```python
from build123d import *

# Parameters (mm, degrees)
SM_BASE_FLANGE_1_DEPTH = 765.5
HOLE_WIZARD_M6_1_D     = 7
HOLE_WIZARD_M5_1_D     = 4.2
HOLE_WIZARD_1_D        = 57


# Sheet-metal steps are written as plain solids
with BuildPart() as part:
    # Sketch 1 → 基体-法兰1 (new, symmetric)
    with BuildSketch(Plane(origin=(0, 0, 0), x_dir=(0, 0, -1), z_dir=(1, 0, 0))):
        with BuildLine():
            Line((0, 0), (0, 17.5))
            ThreePointArc((0, 17.5), (0.732233047, 19.267766953), (2.5, 20))
            Line((2.5, 20), (119, 20))
            ThreePointArc((119, 20), (119.707106781, 20.292893219), (120, 21))
            Line((120, 21), (120, 30))
            Line((120, 30), (121.5, 30))
            Line((121.5, 30), (121.5, 21))
            ThreePointArc((121.5, 21), (120.767766953, 19.232233047), (119, 18.5))
            Line((119, 18.5), (2.5, 18.5))
            ThreePointArc((2.5, 18.5), (1.792893219, 18.207106781), (1.5, 17.5))
            Line((1.5, 17.5), (1.5, 0))
            Line((1.5, 0), (0, 0))
        make_face()
    extrude(amount=SM_BASE_FLANGE_1_DEPTH, both=True)

    # M6 间隙孔1 (through all)
    with Locations(Plane(origin=(0, 0, -1.5), x_dir=(-1, 0, 0), z_dir=(0, 0, -1))):
        with Locations((-650, 8), (0, 8), (650, 8)):
            Hole(HOLE_WIZARD_M6_1_D / 2)

    # M5 螺纹孔1 (through all)
    with Locations(Plane(origin=(0, 20, 0), x_dir=(1, 0, 0), z_dir=(0, 1, 0))):
        with Locations((645.5, 36), (623, 36), (623, 101), (645.5, 101)):
            Hole(HOLE_WIZARD_M5_1_D / 2)

    # 孔1 (through all)
    with Locations(Plane(origin=(0, 20, 0), x_dir=(1, 0, 0), z_dir=(0, 1, 0))):
        with Locations((730.5, 68.5)):
            Hole(HOLE_WIZARD_1_D / 2)


solid = part.part
```
Could you check a few things on this model? Use its own coordinates, in mm. Coordinates: 2 decimals unless noted, no trailing zeros. Write each loop counter-clockwise with the first axis right and the second up, starting at its lowest first coordinate (ties: lowest second). Pieces come first, ordered by that corner, then holes. Notation, with made-up numbers: (72, 36) - (116, 36) arc R12 ccw to (116, 59) - close; hole circle Ø1 at (18.5, 77). An arc over 180 degrees is marked (long way). Use a Markdown table: item, result.
Q1. Please list where these lines run through material, in increasing order: L1, parallel to X at y = 19.4, z = -36; L2, parallel to Z at x = 645.5, y = 19.65; L3, parallel to X at y = 18.85, z = -68.5.
Geometry check:
| item | result |
|---|---|
| L1 | x = -765.5 to 620.9, 625.1 to 643.4, 647.6 to 765.5 |
| L2 | z = -121.1 to -103.1, -98.9 to -38.1, -33.9 to -1.22 |
| L3 | x = -765.5 to 702, 759 to 765.5 |
Q2. Imagine slicing it at C-C (x = 207.5). List the corners of the cut face in (y, z) for me, and give its area (3 significant figures).
Geometry check:
| item | result |
|---|---|
| outline | (0, -1.5) - (17.5, -1.5) arc R1 cw to (18.5, -2.5) - (18.5, -119) arc R2.5 ccw to (21, -121.5) - (30, -121.5) - (30, -120) - (21, -120) arc R1 cw to (20, -119) - (20, -2.5) arc R2.5 ccw to (17.5, 0) - (0, 0) - close |
| area | 223 mm2 |
Q3. I'm going to push flat-ended pins straight in: pin 1 Ø3 at (x, z) = (48, -21) entering from -Y; pin 2 Ø2 at (x, z) = (147, -89) entering from +Y; pin 3 Ø1.5 at (x, y) = (-110.5, 21.5) entering from +Z. Where does each tip first touch, or does it pass through?
Geometry check:
| item | result |
|---|---|
| pin 1 | stops at y = 18.5 |
| pin 2 | stops at y = 20 |
| pin 3 | stops at z = -119.97 |
Q4. Imagine slicing it at B-B (z = -68.5). List the corners of the cut face in (x, y) for me, and give its area (3 significant figures).
Geometry check:
| item | result |
|---|---|
| outline | (-765.5, 18.5) - (702, 18.5) - (702, 20) - (-765.5, 20) - close; (759, 18.5) - (765.5, 18.5) - (765.5, 20) - (759, 20) - close |
| area | 2,210 mm2 |
Q5. Imagine slicing it at A-A (x = 730.5). List the corners of the cut face in (y, z) for me.
Geometry check:
| item | result |
|---|---|
| outline | (0, -1.5) - (17.5, -1.5) arc R1 cw to (18.5, -2.5) - (18.5, -40) - (20, -40) - (20, -2.5) arc R2.5 ccw to (17.5, 0) - (0, 0) - close; (18.5, -119) arc R2.5 ccw to (21, -121.5) - (30, -121.5) - (30, -120) - (21, -120) arc R1 cw to (20, -119) - (20, -97) - (18.5, -97) - close |
Q6. Thinking about a two-plate mould opening in X: for faces 1 (the flat face through (11, 20, -60)), 2 (the flat face through (765.5, 19.5, -61)), 3 (the flat face through (-765.5, 19.5, -61)), 4 (the cylindrical face through (758.972, 19.239, -69.753)), which applies, +X half, -X half, draft (parallel to the pull), parting line (faces both ways), or undercut?
Geometry check:
| item | result |
|---|---|
| face 1 | draft |
| face 2 | +X half |
| face 3 | -X half |
| face 4 | undercut |
